Design review of the part built by this model. Coordinates are the model's own, in mm. Face numbers are marked on the shaded views. Round coordinates to 2 decimals unless told otherwise and drop trailing zeros. Loops run counter-clockwise (first coordinate to the right, second up) from the corner with the lowest first, then second, coordinate; pieces in that order, holes last. Notation, with made-up numbers: (80, 71.25) - (87, 71.25) arc R23 cw to (87, 103.25) - close; hole circle Ø7 at (5, 58.5). An arc over 180 degrees is marked (long way). Use one line per item in the form item = value. Start each with the question number.
(1) For pin 1 (4 mm diameter, centred on y = 78, z = 13.5, fed in from -X); pin 2 (0.6 mm diameter, centred on x = -2, y = -1, fed in from +Z); pin 3 (3 mm diameter, centred on x = -1, y = 60, fed in from +Z), all flat-tipped, find the tip position at first contact; note any pin that passes through.
(2) We need section C-C, the plane z = 3.5. Write out the cut boundary in (x, y).
(3) We need section A-A, the plane x = -2.15. Write out the cut boundary in (y, z).
(4) We need section B-B, the plane y = 78. Write out the cut boundary in (x, z), then the cut area to 3 significant figures.
(5) Wall thickness on probe 1 along Z at (x, y) = (-1.55, 46.5); probe 2 along Y at (x, z) = (-2.35, -14); probe 3 along X at (y, z) = (31.5, 19.5): over which ranges is each line inside the solid? List them lowest first. Write a range as [from, to].
(6) The part is to be moulded in two halves that separate along Z. For the marked faces 1 and 2, say which applies: released by +Z, released by -Z, zero draft, split by the parting line, or undercut.
from build123d import *

# Parameters (mm, degrees)
BOSS_EXTRUDE1_DEPTH = 105
SKETCH2_W           = 5.2
SKETCH2_H           = 34.4
BOSS_EXTRUDE2_DEPTH = 1.2
SKETCH3_W           = 5.2
SKETCH3_H           = 34.4
BOSS_EXTRUDE3_DEPTH = 1.2
CUT_EXTRUDE1_REACH  = 110.369
SKETCH4_W           = 3
SKETCH4_H           = 3
CHAMFER1_SIZE       = 1


with BuildPart() as part:
    # Sketch1 → Boss-Extrude1 (new body)
    with BuildSketch(Plane(origin=(0, 0, 0), x_dir=(1, 0, 0), z_dir=(0, 1, 0))):
        Polygon((0, -16), (0, 16), (-4, 16), (-4, 17.2), (1.2, 17.2), (1.2, -17.2), (1.2, -21.2), (0, -21.2), (0, -17.2), (-4, -17.2), (-4, -16), align=None)
    extrude(amount=BOSS_EXTRUDE1_DEPTH)

    # Sketch2 → Boss-Extrude2 (add)
    with BuildSketch(Plane(origin=(0, 105, 0), x_dir=(1, 0, 0), z_dir=(0, 1, 0))):
        with Locations((-1.4, 0)):
            Rectangle(SKETCH2_W, SKETCH2_H)
    extrude(amount=BOSS_EXTRUDE2_DEPTH)

    # Sketch3 → Boss-Extrude3 (add)
    with BuildSketch(Plane.XZ):
        with Locations((-1.4, 0)):
            Rectangle(SKETCH3_W, SKETCH3_H)
    extrude(amount=BOSS_EXTRUDE3_DEPTH)

    # Sketch4 → Cut-Extrude1 (cut, up to next)
    with BuildSketch(Plane(origin=(0, 0, 0), x_dir=(1, 0, 0), z_dir=(0, 1, 0)), mode=Mode.PRIVATE) as cut_extrude1_sk1:
        with Locations((-1.5, -11)):
            Rectangle(SKETCH4_W, SKETCH4_H)
    cut_extrude1_tool1 = extrude(cut_extrude1_sk1.sketch, amount=-CUT_EXTRUDE1_REACH, mode=Mode.PRIVATE) & part.part
    # Sketch4 → Cut-Extrude1 (cut, up to next)
    with BuildSketch(Plane(origin=(0, 0, 0), x_dir=(1, 0, 0), z_dir=(0, 1, 0)), mode=Mode.PRIVATE) as cut_extrude1_sk2:
        with Locations((-1.5, -3.666666667)):
            Rectangle(SKETCH4_W, SKETCH4_H)
    cut_extrude1_tool2 = extrude(cut_extrude1_sk2.sketch, amount=-CUT_EXTRUDE1_REACH, mode=Mode.PRIVATE) & part.part
    # Sketch4 → Cut-Extrude1 (cut, up to next)
    with BuildSketch(Plane(origin=(0, 0, 0), x_dir=(1, 0, 0), z_dir=(0, 1, 0)), mode=Mode.PRIVATE) as cut_extrude1_sk3:
        with Locations((-1.5, 3.666666667)):
            Rectangle(SKETCH4_W, SKETCH4_H)
    cut_extrude1_tool3 = extrude(cut_extrude1_sk3.sketch, amount=-CUT_EXTRUDE1_REACH, mode=Mode.PRIVATE) & part.part
    # Sketch4 → Cut-Extrude1 (cut, up to next)
    with BuildSketch(Plane(origin=(0, 0, 0), x_dir=(1, 0, 0), z_dir=(0, 1, 0)), mode=Mode.PRIVATE) as cut_extrude1_sk4:
        with Locations((-1.5, 11)):
            Rectangle(SKETCH4_W, SKETCH4_H)
    cut_extrude1_tool4 = extrude(cut_extrude1_sk4.sketch, amount=-CUT_EXTRUDE1_REACH, mode=Mode.PRIVATE) & part.part
    add(cut_extrude1_tool1.solids().sort_by_distance((-1.5, 0, 11))[0], mode=Mode.SUBTRACT)
    add(cut_extrude1_tool2.solids().sort_by_distance((-1.5, 0, 3.666667))[0], mode=Mode.SUBTRACT)
    add(cut_extrude1_tool3.solids().sort_by_distance((-1.5, 0, -3.666667))[0], mode=Mode.SUBTRACT)
    add(cut_extrude1_tool4.solids().sort_by_distance((-1.5, 0, -11))[0], mode=Mode.SUBTRACT)

    # Chamfer1
    # the kernel refuses this chamfer: 1 mm, written as the material it takes off along each edge
    with BuildSketch(Plane(origin=(0, -2.571682988, 21.2), x_dir=(-0.02749587661058639, 0, -0.9996219169112968), z_dir=(0, 1, 0))) as chamfer1_piece_1:
        Polygon((CHAMFER1_SIZE * 0.999621916911, -CHAMFER1_SIZE * 0.0274958766106), (-CHAMFER1_SIZE * 0.0274958766106, -CHAMFER1_SIZE * 0.999621916911), (0, 0), align=None)
    extrude(amount=110.143365976, mode=Mode.SUBTRACT)
    with BuildSketch(Plane(origin=(1.2, -2.571682988, 21.2), x_dir=(0.027495876610586077, 0, -0.9996219169112968), z_dir=(0, 1, 0))) as chamfer1_piece_2:
        Polygon((CHAMFER1_SIZE * 0.999621916911, CHAMFER1_SIZE * 0.0274958766106), (-CHAMFER1_SIZE * 0.0274958766106, CHAMFER1_SIZE * 0.999621916911), (0, 0), align=None)
    extrude(amount=110.143365976, mode=Mode.SUBTRACT)


solid = part.part
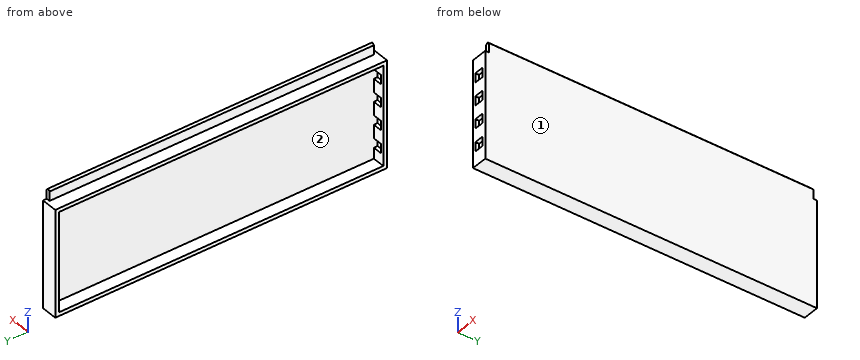
Data:
q1.pin_1 = 0
q1.pin_2 = 17.2
q1.pin_3 = 20.7
q2.outline = (-4, -1.2) - (-3, -1.2) - (-3, 0) - (-4, 0) - close; (-4, 105) - (0, 105) - (0, -1.2) - (1.2, -1.2) - (1.2, 106.2) - (-4, 106.2) - close
q3.outline = (-1.2, -17.2) - (106.2, -17.2) - (106.2, 17.2) - (-1.2, 17.2) - (-1.2, 12.5) - (0, 12.5) - (0, 16) - (105, 16) - (105, -16) - (0, -16) - (0, -12.5) - (-1.2, -12.5) - close; (-1.2, -9.5) - (0, -9.5) - (0, -5.17) - (-1.2, -5.17) - close; (-1.2, -2.17) - (0, -2.17) - (0, 2.17) - (-1.2, 2.17) - close; (-1.2, 5.17) - (0, 5.17) - (0, 9.5) - (-1.2, 9.5) - close
q4.outline = (-4, -17.2) - (1.2, -17.2) - (1.2, 20.2) - (0.6, 20.8) - (0, 20.2) - (0, 17.2) - (-4, 17.2) - (-4, 16) - (0, 16) - (0, -16) - (-4, -16) - close
q4.area = 54.8 mm^2
q5.probe_1 = [-17.2, -16], [16, 17.2]
q5.probe_2 = [-1.2, 0], [105, 106.2]
q5.probe_3 = [0, 1.2]
q6.face_1 = zero draft
q6.face_2 = undercut
